from build123d import *

# Parameters (mm, degrees)
BOSS_EXTRUDE1_DEPTH = 28
SHELL1_T            = -2


with BuildPart() as part:
    # Sketch1 → Boss-Extrude1 (new body)
    with BuildSketch(Plane.XY):
        with BuildLine():
            Line((38, -220), (38, -180.544315889))
            ThreePointArc((38, -180.544315889), (0, -184.5), (-38, -180.544315889))
            Line((-38, -180.544315889), (-38, -220))
            Line((-38, -220), (38, -220))
        make_face()
    extrude(amount=-BOSS_EXTRUDE1_DEPTH)

    # Shell1
    shell1_openings = [part.faces().sort_by_distance(p)[0] for p in [
        (38, -200.272157945, -14),
        (0, -184.5, -14),
        (0, -201.574740198, -28),
        (-38, -200.272157945, -14),
    ]]
    offset(amount=SHELL1_T, openings=shell1_openings, kind=Kind.INTERSECTION)


solid = part.part
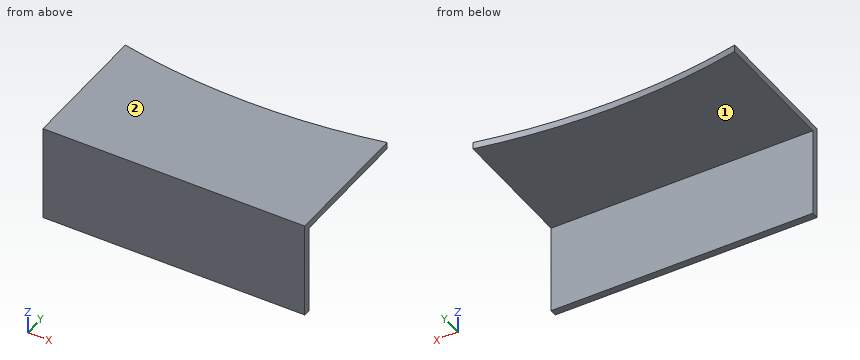
Geometry: final body of the model. Coordinates: model frame, mm. Face numbers are marked on the shaded views. A direction names the side the tool comes from. Give positions to 0.01 mm unless a question says otherwise; leave off trailing zeros. Loops run counter-clockwise (first coordinate to the right, second up) from the corner with the lowest first, then second, coordinate; pieces in that order, holes last. Notation, with made-up numbers: M 3,74 L 48,74 A19 ccw 48,93 Z; hole C 15.25,74.25 d5. An arc over 180 degrees is marked long. Put each result on its own line as item: value. Start each with the question number.
1) Ray query, line 1 along Z through (x, y) = (-5.5, -201.5); line 2 along Y through (x, z) = (-0.5, -5.5). Return the intervals inside material, ascending.
2) Contact query for flat-ended pins moving along their axis: pin 1 (13 mm diameter, centred on x = 3, z = -15, fed in from +Y); pin 2 (18.5 mm diameter, centred on x = 13, y = -207, fed in from -Z); pin 3 (2 mm diameter, centred on x = 25, y = -196.5, fed in from +Z). Output: stop coordinate, or through.
3) Cut plane B-B (y = -204.5). Output: boundary loops of the cut face in (x, z), then the cut area to 3 significant figures.
4) Cut plane D-D (x = 9). Output: boundary loops of the cut face in (y, z).
5) Cut plane A-A (x = 18). Output: boundary loops of the cut face in (y, z).
6) Access query for the marked faces 1 and 2. Directions: +Z, -Z, +X, -X, +Y, -Y. A direction counts if a zero-diameter tool reaches every point of the face in a straight line with its end or side. Return the directions, or none.
7) Cut plane C-C (z = -24.25). Output: boundary loops of the cut face in (x, y), then the cut area to 3 significant figures.
Verdict:
1. line 1: -2 to 0
1. line 2: -220 to -218
2. pin 1: y = -218
2. pin 2: z = -2
2. pin 3: z = 0
3. outline: M -38,-2 L 38,-2 L 38,0 L -38,0 Z
3. area: 152 mm2
4. outline: M -220,-28 L -218,-28 L -218,-2 L -184.28,-2 L -184.28,0 L -220,0 Z
5. outline: M -220,-28 L -218,-28 L -218,-2 L -183.62,-2 L -183.62,0 L -220,0 Z
6. face 1: -Z, +X, -X, +Y
6. face 2: +Z, +X, -X, +Y, -Y
7. outline: M -38,-220 L 38,-220 L 38,-218 L -38,-218 Z
7. area: 152 mm2
